from build123d import *

# Parameters (mm, degrees)
SKETCH1_R           = 1.5
BOSS_EXTRUDE1_DEPTH = 3


with BuildPart() as part:
    # Sketch1 → Boss-Extrude1 (new body)
    with BuildSketch(Plane(origin=(0, 0, 0), x_dir=(1, 0, 0), z_dir=(0, 1, 0))):
        Polygon((-47.380002118, 7.413403038), (-47.380002118, 4.413403038), (-55.380002118, 4.413403038), (-55.380002118, 0.413403038), (-58.380002118, 0.413403038), (-58.380002118, -4.586596962), (-55.380002118, -4.586596962), (-55.380002118, -9.086596962), (-15.820002118, -9.086596962), (-4.330002118, 2.403403038), (-4.330002118, 4.413403038), (-37.380002118, 4.413403038), (-37.380002118, 7.413403038), align=None)
        with Locations((-36.380002118, -3.586596962)):
            Circle(SKETCH1_R, mode=Mode.SUBTRACT)
    extrude(amount=BOSS_EXTRUDE1_DEPTH)


solid = part.part
The model under review builds one solid part; all positions refer to its coordinate system, in mm. A direction names the side the tool comes from. Give positions to 0.01 mm unless a question says otherwise; leave off trailing zeros. Write each loop counter-clockwise with the first axis right and the second up, starting at its lowest first coordinate (ties: lowest second). Pieces come first, ordered by that corner, then holes. Notation, with made-up numbers: M 62.5,11 L 105.5,11 A11 cw 105.5,23 Z; hole C 43.5,-27 d11. An arc over 180 degrees is marked long. One line per question, with ' | ' between items. Start each with the question number.
Item 1: For faces 4 (the flat face through (-57, 1, -0.413)), 5 (the flat face through (-37.38, 1, -6)), 6 (the flat face through (-55.38, 1, 7)), list the 3-axis set-ups (+Z, -Z, +X, -X, +Y, -Y) from which the entire face can be reached by the end or side of a thin tool; tool diameter is ignored.
Item 2: Wall thickness on line 1 (X direction, y = 0.9, z = -6.5); line 2 (Z direction, x = -22, y = 1.1); line 3 (X direction, y = 2.85, z = -3): over which ranges is each line inside the solid? List them lowest first. Write a range as from..to.
Item 3: Draft analysis for pull direction X (two halves, no side actions). For faces 1 (the flat face through (-10.155, 1.479, 3.422)), 2 (the flat face through (-47.38, 1, -6)), 3 (the cylindrical face through (-37.486, 1.479, 2.573)), state which applies: released by +X, released by -X, zero draft, split by the parting line, or undercut.
Item 4: We need section A-A on y = 0.5. Write out the cut boundary in (x, z).
Item 5: For pin 1 (1.5 mm diameter, centred on x = -50.5, y = 2, fed in from -Z); pin 2 (6 mm diameter, centred on x = -51, z = 4.5, fed in from -Y), all flat-tipped, find the tip position at first contact; note any pin that passes through.
Item 6: We need section B-B on x = -54. Write out the cut boundary in (y, z), plus the area to 3 significant figures.
Item 7: We need section C-C on z = -3. Write out the cut boundary in (x, y).
Results found:
1) face 4: -Z, -X, +Y, -Y | face 5: -Z, +X, +Y, -Y | face 6: +Z, -X, +Y, -Y
2) line 1: x = -47.38..-37.38 | line 2: z = -4.41..9.09 | line 3: x = -55.38..-4.33
3) face 1: released by +X | face 2: released by -X | face 3: undercut
4) outline: M -58.38,-0.41 L -55.38,-0.41 L -55.38,-4.41 L -47.38,-4.41 L -47.38,-7.41 L -37.38,-7.41 L -37.38,-4.41 L -4.33,-4.41 L -4.33,-2.4 L -15.82,9.09 L -55.38,9.09 L -55.38,4.59 L -58.38,4.59 Z; hole C -36.38,3.59 d3
5) pin 1: stops at z = -4.41 | pin 2: stops at y = 0
6) outline: M 0,-4.41 L 3,-4.41 L 3,9.09 L 0,9.09 Z | area: 40.5 mm2
7) outline: M -55.38,0 L -4.33,0 L -4.33,3 L -55.38,3 Z
